Geometry check sheet. Reference: drawing and pictorial views, mm from the part's lowest x, y, z. Round coordinates to 2 decimals unless told otherwise and drop trailing zeros. Write each loop counter-clockwise with the first axis right and the second up, starting at its lowest first coordinate (ties: lowest second). Pieces come first, ordered by that corner, then holes. Notation, with made-up numbers: (40, 12) - (86, 12) arc R28 cw to (86, 40) - close; hole circle Ø5 at (79, 58.25). An arc over 180 degrees is marked (long way). Return JSON: item names as keys, results as strings.
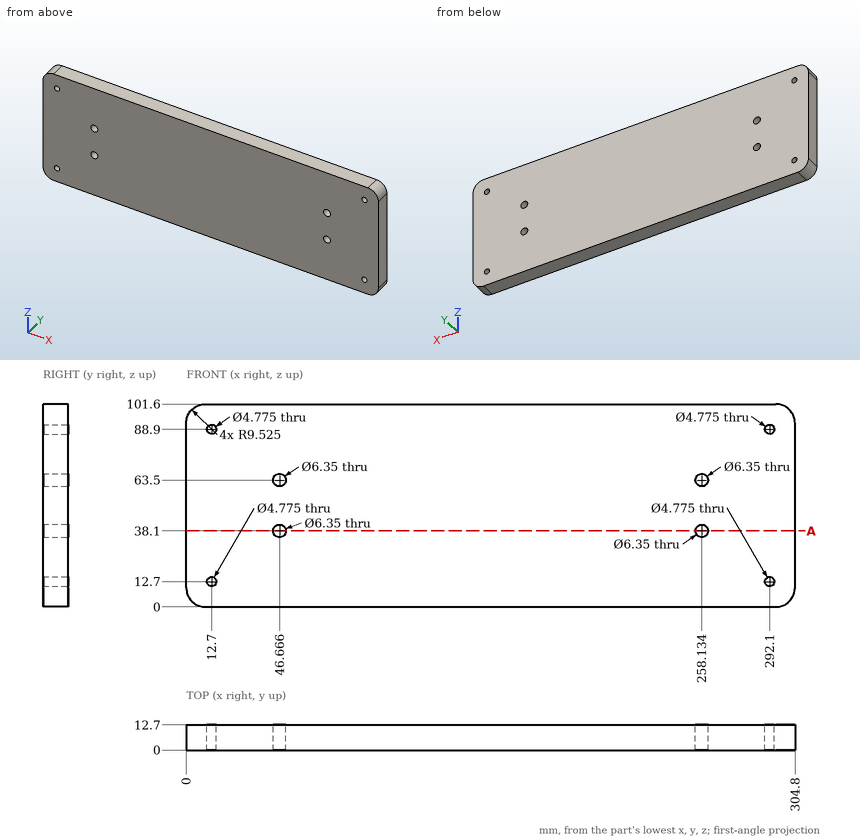
(1) Material ranges on line 1 along Z through (x, y) = (292.1, 6.25); line 2 along X through (y, z) = (2.75, 88); line 3 along X through (y, z) = (8, 91) (1 decimal), recorded low to high. Write a range as [from, to].
Response values:
{"line 1": "z = [0, 10.31], [15.09, 86.51], [91.29, 101.6]", "line 2": "x = [0, 10.49], [14.91, 289.89], [294.31, 304.8]", "line 3": "x = [0, 11.6], [13.8, 291], [293.2, 304.8]"}
(2) Section check A-A, the plane z = 38.1. Enter the section's corners in (x, y), plus the area to 3 significant figures.
Response values:
{"outline": "(0, 0) - (43.49, 0) - (43.49, 12.7) - (0, 12.7) - close; (49.84, 0) - (254.96, 0) - (254.96, 12.7) - (49.84, 12.7) - close; (261.31, 0) - (304.8, 0) - (304.8, 12.7) - (261.31, 12.7) - close", "area": "3,710 mm^2"}
(3) Gauge pin test, flat end, axial feed: pin 1 (5 mm diameter, centred on x = 46.67, z = 38.1, fed in from +Y). Record the tip position at first contact, or that the pin passes through.
Response values:
{"pin 1": "passes through"}
